Work out the finished part from the listing and answer in its coordinate system (mm). Coordinates: 2 decimals unless noted, no trailing zeros. Write each loop counter-clockwise with the first axis right and the second up, starting at its lowest first coordinate (ties: lowest second). Pieces come first, ordered by that corner, then holes. Notation, with made-up numbers: (-34.5, 75) - (17.5, 75) arc R32 cw to (17.5, 114) - close; hole circle Ø6 at (47, 68). An arc over 180 degrees is marked (long way). Answer as a JSON object with one key per item and string values. Group by question number.
from build123d import *

# Parameters (mm, degrees)
F0_W     = 80
F0_H     = 20
F2_DEPTH = 10
F1_R     = 6.5
F3_DEPTH = 10
F4_R     = 3.5
F5_DEPTH = 20


with BuildPart() as f2:
    # F0 (on Front) → F2 (new body, symmetric)
    with BuildSketch(Plane.XZ):
        Rectangle(F0_W, F0_H)
    extrude(amount=F2_DEPTH, both=True)

    # F1 (on Front) → F3 (cut, symmetric)
    with BuildSketch(Plane.XZ):
        with Locations((-28.001357, 10.137838)):
            Circle(F1_R)
        with Locations((28.001095, 10.123801)):
            Circle(F1_R)
    extrude(amount=F3_DEPTH, both=True, mode=Mode.SUBTRACT)

    # F4 (on Top) → F5 (cut, symmetric)
    with BuildSketch(Plane.XY):
        with Locations((-27.499896, 0)):
            Circle(F4_R)
        with Locations((27.499916, 0)):
            Circle(F4_R)
    extrude(amount=F5_DEPTH, both=True, mode=Mode.SUBTRACT)


solid = f2.part
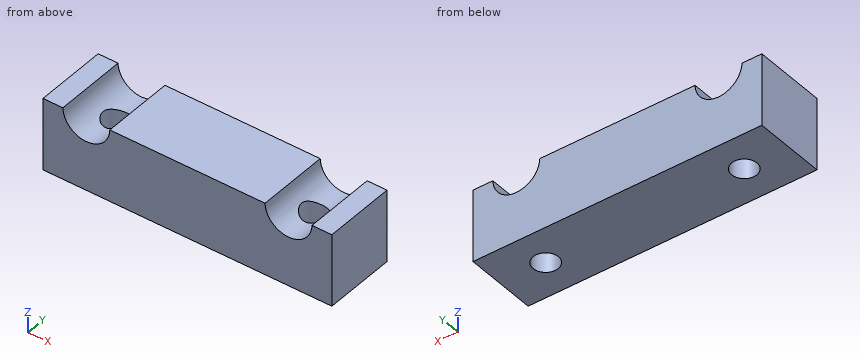
Q1. Section D-D on y = 7 is taken. Determine the outline of the cut face in (x, z), plus the area to 3 significant figures.
Q2. Consider L1, parallel to X at y = 0, z = -4.5; L2, parallel to X at y = -1, z = -6.25; L3, parallel to Z at x = 28, y = -8.5. Determine where each line is inside the solid, lowest interval first. Write a range as from..to.
Q3. Section A-A on y = 2.25 is taken. Determine the outline of the cut face in (x, z).
Q4. Section C-C on z = 2.75 is taken. Determine the outline of the cut face in (x, y), plus the area to 3 significant figures.
Q5. Section B-B on z = 8 is taken. Determine the outline of the cut face in (x, y).
Numbers:
{
 "1": {"outline": "(-40, -10) - (40, -10) - (40, 10) - (34.5, 10) arc R6.5 cw to (21.5, 10) - (-21.5, 10) arc R6.5 cw to (-34.5, 10) - (-40, 10) - close", "area": "1,470 mm²"},
 "2": {"L1": "x = -40..-31, -24..24, 31..40", "L2": "x = -40..-30.85, -24.15..24.15, 30.85..40", "L3": "z = -10..3.62"},
 "3": {"outline": "(-40, -10) - (-30.18, -10) - (-30.18, 4.01) arc R6.5 cw to (-34.5, 10) - (-40, 10) - close; (-24.82, -10) - (24.82, -10) - (24.82, 4.46) arc R6.5 cw to (21.5, 10) - (-21.5, 10) arc R6.5 cw to (-24.82, 4.47) - close; (30.18, -10) - (40, -10) - (40, 10) - (34.5, 10) arc R6.5 cw to (30.18, 4) - close"},
 "4": {"outline": "(-40, -10) - (40, -10) - (40, 10) - (-40, 10) - close; hole circle Ø7 at (-27.5, 0); hole circle Ø7 at (27.5, 0)", "area": "1,520 mm²"},
 "5": {"outline": "(-40, -10) - (-34.14, -10) - (-34.14, 10) - (-40, 10) - close; (-21.86, -10) - (21.86, -10) - (21.86, 10) - (-21.86, 10) - close; (34.14, -10) - (40, -10) - (40, 10) - (34.14, 10) - close"}
}
